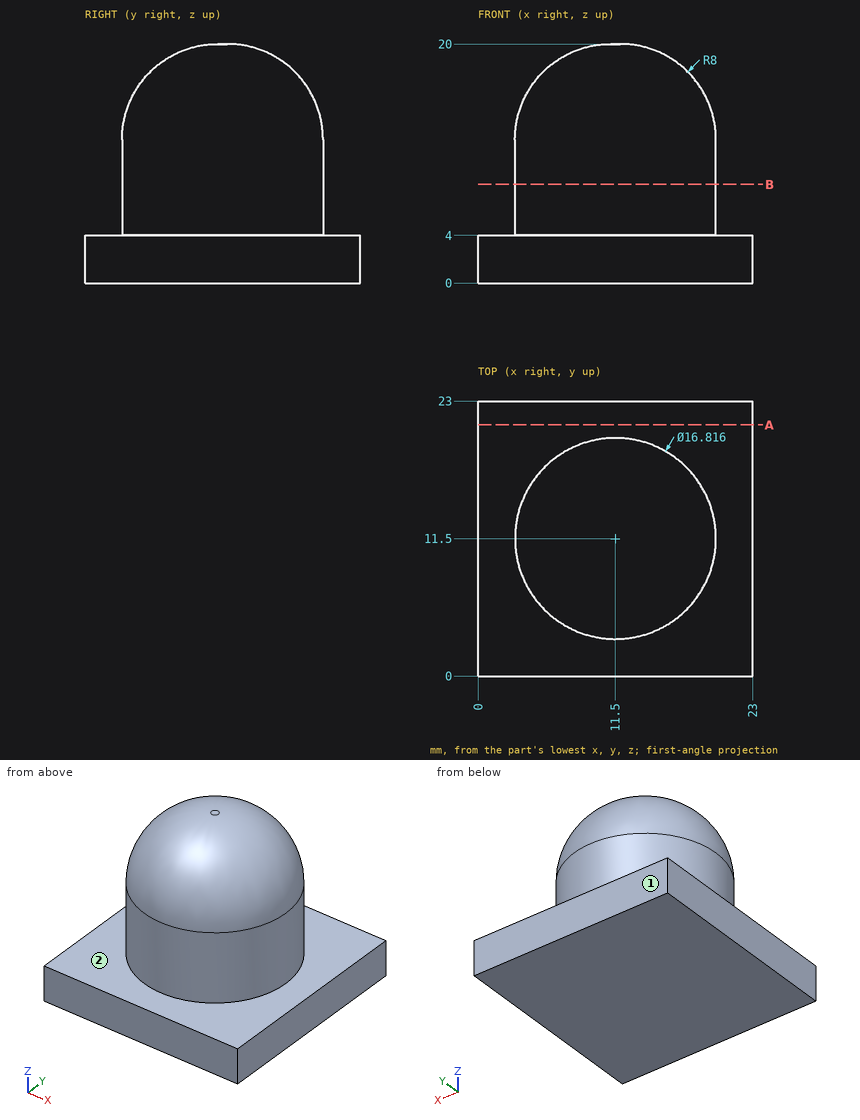
The figure shows three views and two pictorial views of one solid part (mm, origin at its lowest corner). Answer the questions. A direction names the side the tool comes from. Round coordinates to 2 decimals unless told otherwise and drop trailing zeros. Write each loop counter-clockwise with the first axis right and the second up, starting at its lowest first coordinate (ties: lowest second). Pieces come first, ordered by that corner, then holes. Notation, with made-up numbers: (85.5, 67.25) -> (92.5, 67.25) arc R13 ccw to (92.5, 73.25) -> close; hole circle Ø7 at (3.5, -31.5). An arc over 180 degrees is marked (long way). Answer as a JSON object with one key per item and string values. Group by question number.
Q1. Straight lines are drawn through the part: line 1 along Z through (x, y) = (16.25, 3); line 2 along X through (y, z) = (9, 17.5) (1 decimal); line 3 along Y through (x, z) = (18.75, 9) (1 decimal). For each, find the intervals that lie inside material, in ascending order.
Q2. Which of the six approach directions +Z, -Z, +X, -X, +Y, -Y give full straight-line access (tool end or side, diameter ignored) to the marked faces 1 and 2?
Q3. Section B-B (z = 8.25) is taken. Write down the section's boundary in (x, y), plus the area to 3 significant figures.
Q4. Each of these flat-tipped pins is pushed along its axis until it touches: pin 1 Ø2 at (y, z) = (18, 8.5) entering from +X; pin 2 Ø1 at (y, z) = (13, 16.5) entering from +X; pin 3 Ø6 at (x, z) = (8.5, 12.5) entering from -Y. Where does it stop, or does it pass through?
Q5. Section A-A (y = 21) is taken. Write down the section's boundary in (x, z).
Check values:
{
 "1": {"line 1": "0 to 4", "line 2": "5.8 to 17.2", "line 3": "7.2 to 15.8"},
 "2": {"face 1": "+Z, -Z, +X, -X, +Y", "face 2": "+Z"},
 "3": {"outline": "circle Ø16.82 at (11.5, 11.5)", "area": "222 mm^2"},
 "4": {"pin 1": "x = 17.86", "pin 2": "x = 18.7", "pin 3": "y = 3.09"},
 "5": {"outline": "(0, 0) -> (23, 0) -> (23, 4) -> (0, 4) -> close"}
}
